Here's how the part is built. I have some questions about the finished solid (model axes, mm). Give positions to 0.01 mm unless a question says otherwise; leave off trailing zeros. Loops run counter-clockwise (first coordinate to the right, second up) from the corner with the lowest first, then second, coordinate; pieces in that order, holes last. Notation, with made-up numbers: (73, -27) - (104, -27) arc R24 ccw to (104, 10) - close; hole circle Ø5 at (45.5, 23.25). An arc over 180 degrees is marked (long way). Use one line per item in the form item = value.
from build123d import *

# Parameters (mm, degrees)
F1_DEPTH = 1


# Not quite as in the source:
# - ends of sketch curves that miss each other by under 0.0002 mm in the source are joined


with BuildPart() as f1:
    # F0 (on Top) → F1 (new body)
    with BuildSketch(Plane.XY):
        Polygon((84.760502, 99.838331), (84.760502, 65.532372), (84.760502, 29.104707), (143.7776135408, 28.8903586668), (163.977411, 28.886699), (163.977411, 28.816993624), (164.3435, 28.815664), (164.3435, 27.535789), (163.977411, 27.535789), (163.977411, 27.386699), (85.0591829073, 27.400996887), (84.3979659422, -40.0634812645), (145.310694, -40.074967), (145.31063, -41.574967), (84.3837574867, -41.5131809608), (84.0646295035, -74.0740558181), (120.630506, -74.117418), (120.630358, -75.617418), (84.0482665226, -75.7435834112), (84.760502, -91.880651), (93.474501, -91.537649), (107.070486, -89.99767), (120.241516, -87.578631), (132.799484, -84.348639), (144.519505, -80.423663), (155.382483, -75.955654), (165.369519, -71.08065), (242.942492, 24.705363), (243.065503, 133.841338), (165.369519, 229.998345), (155.382483, 234.875351), (144.519505, 239.356344), (132.799484, 243.272341), (120.241516, 246.491352), (107.059515, 248.919369), (93.474501, 250.452351), (84.760502, 250.797334), (84.760502, 234.60194), (84.7707435172, 234.6018600186), (84.770746, 234.626524), (121.161056, 234.620025), (121.160905, 233.120025), (121.132491, 233.1200300745), (121.132491, 233.026024), (85.060504, 233.026024), (84.910536, 200.618297), (145.27452, 200.708488), (145.27452, 199.072799), (85.060504, 199.072799), (84.760502, 168.454341), (84.760502, 132.02771), (164.127413, 131.611891), (164.127413, 130.111891), (84.910503, 130.126243), (84.7605566, 99.8493557296), align=None)
    extrude(amount=F1_DEPTH)


solid = f1.part
(1) If we section it at B-B (x = 128): List the corners of the cut face in (y, z) for me, plus the area to 3 significant figures.
Geometry says:
outline = (-85.58, 0) - (-41.56, 0) - (-41.56, 1) - (-85.58, 1) - close; (-40.07, 0) - (27.39, 0) - (27.39, 1) - (-40.07, 1) - close; (28.95, 0) - (130.12, 0) - (130.12, 1) - (28.95, 1) - close; (131.8, 0) - (199.07, 0) - (199.07, 1) - (131.8, 1) - close; (200.68, 0) - (244.5, 0) - (244.5, 1) - (200.68, 1) - close
area = 324 mm²
(2) For P1, Ø0.5, axis at x = 155, z = 0.5, coming from the -Y side; P2, Ø1, axis at x = 132, y = 184.5, coming from the -Z side; P3, Ø0.5, axis at x = 109.5, z = 0.5, coming from the -Y side, each with a flat end and sliding along its axis, tell me the tip position at first contact or that it passes through.
Geometry says:
P1 = -76.22
P2 = 0
P3 = -89.6
(3) If we section it at C-C (x = 160): List the corners of the cut face in (y, z) for me.
Geometry says:
outline = (-73.7, 0) - (27.39, 0) - (27.39, 1) - (-73.7, 1) - close; (28.89, 0) - (130.11, 0) - (130.11, 1) - (28.89, 1) - close; (131.63, 0) - (232.62, 0) - (232.62, 1) - (131.63, 1) - close
(4) If I drill on probe 1 along Y at (x, z) = (153, 0.15); probe 2 along Y at (x, z) = (121.5, 0.8); probe 3 along Y at (x, z) = (154.5, 0.1), over which ranges is the centre line in solid material (lowest first)?
Geometry says:
probe_1 = -76.94 to 27.39, 28.89 to 130.11, 131.67 to 235.86
probe_2 = -87.25 to -41.55, -40.07 to 27.39, 28.97 to 130.12, 131.84 to 199.07, 200.67 to 246.17
probe_3 = -76.32 to 27.39, 28.89 to 130.11, 131.66 to 235.24
(5) If we section it at D-D (y = 174.5): List the corners of the cut face in (x, z) for me.
Geometry says:
outline = (84.82, 0) - (210.21, 0) - (210.21, 1) - (84.82, 1) - close
(6) If we section it at A-A (x = 101): List the corners of the cut face in (y, z) for me, plus the area to 3 significant figures.
Geometry says:
outline = (-90.69, 0) - (-75.69, 0) - (-75.69, 1) - (-90.69, 1) - close; (-74.09, 0) - (-41.53, 0) - (-41.53, 1) - (-74.09, 1) - close; (-40.07, 0) - (27.4, 0) - (27.4, 1) - (-40.07, 1) - close; (29.05, 0) - (130.12, 0) - (130.12, 1) - (29.05, 1) - close; (131.94, 0) - (199.07, 0) - (199.07, 1) - (131.94, 1) - close; (200.64, 0) - (233.03, 0) - (233.03, 1) - (200.64, 1) - close; (234.62, 0) - (249.6, 0) - (249.6, 1) - (234.62, 1) - close
area = 331 mm²
